For this review, take the finished solid that the model builds, in its own axes (mm). Give positions to 0.01 mm unless a question says otherwise; leave off trailing zeros. Write each loop counter-clockwise with the first axis right and the second up, starting at its lowest first coordinate (ties: lowest second). Pieces come first, ordered by that corner, then holes. Notation, with made-up numbers: (6, 12.25) -> (49, 12.25) arc R4 ccw to (49, 18.25) -> close; hole circle Ø6 at (49.25, 83). An arc over 180 degrees is marked (long way). Answer as CSV lines item,"result".
```python
from build123d import *

# Parameters (mm, degrees)
SKETCH1_R           = 5.08
BOSS_EXTRUDE1_DEPTH = 101.6
SKETCH2_R           = 3.175
BOSS_EXTRUDE2_DEPTH = 25.4
SCALE1_SCALE        = 0.66


with BuildPart() as part:
    # Sketch1 → Boss-Extrude1 (new, symmetric)
    with BuildSketch(Plane.XY):
        Circle(SKETCH1_R)
    extrude(amount=BOSS_EXTRUDE1_DEPTH, both=True)

    # Sketch2 → Boss-Extrude2 (add)
    with BuildSketch(Plane.XY.offset(101.6)):
        Circle(SKETCH2_R)
    boss_extrude2 = extrude(amount=BOSS_EXTRUDE2_DEPTH)

    # Mirror1: Boss-Extrude2 across plane
    add(boss_extrude2.mirror(Plane.XY))


with BuildPart() as part_1:
    # Scale1: scaled about (0, 0, 0)
    add(part.part.scale(SCALE1_SCALE))


solid = part_1.part
```
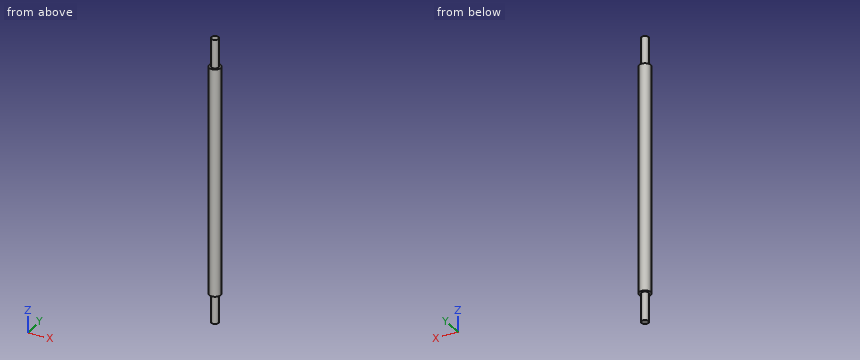
Q1. Add section C-C (z = -70.5). Write out the cut boundary in (x, y), plus the area to 3 significant figures.
Answer block:
outline,"circle Ø4.19 at (0, 0)"
area,"13.8 mm2"
Q2. Clearance check with flat-ended pins moving along their axes: pin 1 (1 mm diameter, centred on x = -1.5, z = 62.5, fed in from -Y); pin 2 (1 mm diameter, centred on y = -1.5, z = 8, fed in from -X); pin 3 (1 mm diameter, centred on x = -2, z = -58.5, fed in from -Y). State where each tip first meets the part, or that it passes through.
Answer block:
pin 1,"stops at y = -3.2"
pin 2,"stops at x = -3.2"
pin 3,"stops at y = -3"
Q3. Add section D-D (z = 31.5). Write out the cut boundary in (x, y), plus the area to 3 significant figures.
Answer block:
outline,"circle Ø6.71 at (0, 0)"
area,"35.3 mm2"
Q4. Add section A-A (x = 0). Write out the cut boundary in (y, z).
Answer block:
outline,"(-3.35, -67.06) -> (-2.1, -67.06) -> (-2.1, -83.82) -> (2.1, -83.82) -> (2.1, -67.06) -> (3.35, -67.06) -> (3.35, 67.06) -> (2.1, 67.06) -> (2.1, 83.82) -> (-2.1, 83.82) -> (-2.1, 67.06) -> (-3.35, 67.06) -> close"
Q5. To check wall thickness, follow probe 1 along X at (y, z) = (0.25, 68.5); probe 2 along Z at (x, y) = (-2, 2); probe 3 along X at (y, z) = (1, -5). State the ranges of each line that lie inside material, in increasing order. Write a range as [from, to].
Answer block:
probe 1,"x = [-2.08, 2.08]"
probe 2,"z = [-67.06, 67.06]"
probe 3,"x = [-3.2, 3.2]"
